Part print with two shaded views. Sizes in mm from the minimum x, y, z corner. Round coordinates to 2 decimals unless told otherwise and drop trailing zeros. Write each loop counter-clockwise with the first axis right and the second up, starting at its lowest first coordinate (ties: lowest second). Pieces come first, ordered by that corner, then holes. Notation, with made-up numbers: (40, 55.5) -> (67, 55.5) arc R25 ccw to (67, 87.5) -> close; hole circle Ø6 at (74.25, 55). An arc over 180 degrees is marked (long way). Answer in a Markdown table with one row per item.
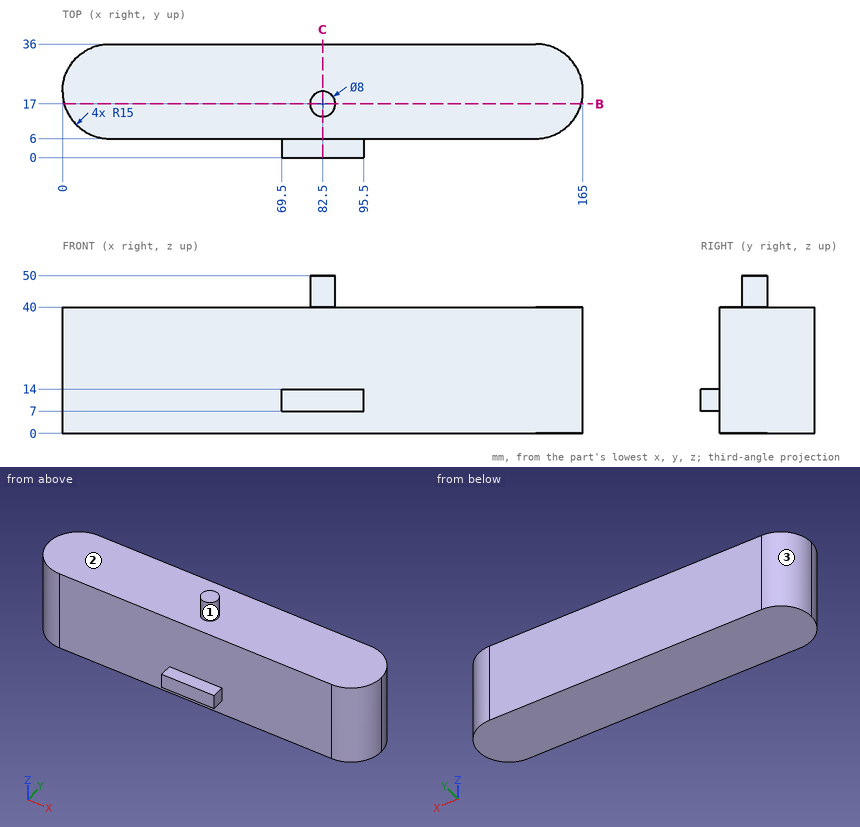
Q1. Saw through at C-C on x = 82.5. Write the cut outline in (y, z).
A:
| item | result |
|---|---|
| outline | (0, 7) -> (6, 7) -> (6, 0) -> (36, 0) -> (36, 40) -> (21, 40) -> (21, 50) -> (13, 50) -> (13, 40) -> (6, 40) -> (6, 14) -> (0, 14) -> close |
Q2. Wall check: line 1 (Z direction, x = 112.5, y = 20.5); line 2 (Y direction, x = 137.5, z = 38); line 3 (X direction, y = 16.5, z = 45.5). Give the ranges that are in metal, low to high. Write a range as [from, to].
A:
| item | result |
|---|---|
| line 1 | [0, 40] |
| line 2 | [6, 36] |
| line 3 | [78.53, 86.47] |
Q3. Saw through at B-B on y = 17. Write the cut outline in (x, z), plus the area to 3 significant figures.
A:
| item | result |
|---|---|
| outline | (0.54, 0) -> (164.46, 0) -> (164.46, 40) -> (86.5, 40) -> (86.5, 50) -> (78.5, 50) -> (78.5, 40) -> (0.54, 40) -> close |
| area | 6,640 mm² |
Q4. Drop flat-ended pins along their axis: P1, Ø12, axis at y = 14, z = 39, coming from the +X side; P2, Ø5, axis at x = 23, z = 18.5, coming from the -Y side; P3, Ø6.5, axis at y = 2, z = 11, coming from the +X side. Give the stop position or say it passes through.
A:
| item | result |
|---|---|
| P1 | x = 164.97 |
| P2 | y = 6 |
| P3 | x = 95.5 |
Q5. Two-plate mould, pull along Y, no slides. Class the marked faces 1, 2 and 3: released by +Y, released by -Y, zero draft, split by the parting line, or undercut.
A:
| item | result |
|---|---|
| face 1 | split by the parting line |
| face 2 | zero draft |
| face 3 | released by +Y |
